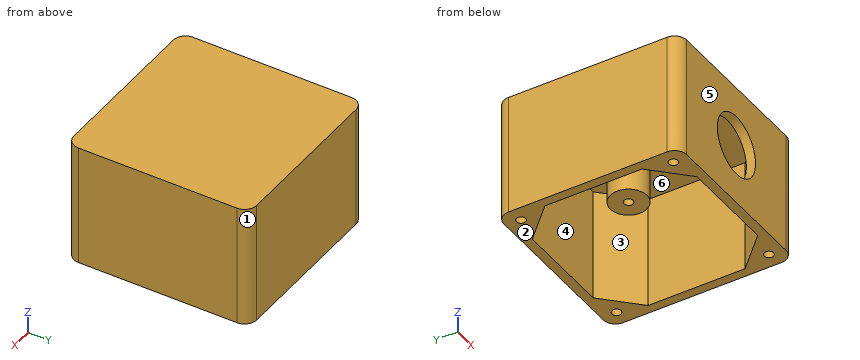
from build123d import *

# Parameters (mm, degrees)
SKETCH014_W     = 30
SKETCH014_H     = 30
PAD008_DEPTH    = 20
POCKET006_DEPTH = 18.5
SKETCH016_R     = 3
PAD009_DEPTH    = 6.5
SKETCH017_R     = 0.75
POCKET007_DEPTH = 5
SKETCH018_R     = 0.75
POCKET008_DEPTH = 15
SKETCH021_R     = 5
POCKET009_DEPTH = 5
FILLET001_R     = 2


with BuildPart() as part:
    # Sketch014 (on Face1 of ReferencePocket001) → Pad008 (new body)
    with BuildSketch(Plane(origin=(0, 0, 0), x_dir=(1, 0, 0), z_dir=(0, 0, -1))):
        with Locations((0, 2.9356231958)):
            Rectangle(SKETCH014_W, SKETCH014_H)
    extrude(amount=PAD008_DEPTH)

    # Sketch015 (on Face6 of Pad008) → Pocket006 (cut)
    with BuildSketch(Plane(origin=(0, 0, -20), x_dir=(1, 0, 0), z_dir=(0, 0, -1))):
        Polygon((-13.5, -5.0288428982), (-13.5, 10.9000892899), (-7.9644660941, 16.4356231958), (7.9644660941, 16.4356231958), (13.5, 10.9000892899), (13.5, -5.0288428982), (7.9644660941, -10.5643768042), (-7.9644660941, -10.5643768042), align=None)
    extrude(amount=-POCKET006_DEPTH, mode=Mode.SUBTRACT)

    # Sketch016 (on Face1 of ReferencePocket001) → Pad009 (join)
    with BuildSketch(Plane(origin=(0, 0, 0), x_dir=(1, 0, 0), z_dir=(0, 0, -1))):
        with Locations((-7, -4.15)):
            Circle(SKETCH016_R)
        with Locations((7, -4.15)):
            Circle(SKETCH016_R)
    extrude(amount=PAD009_DEPTH)

    # Sketch017 (on Face20 of Pad009) → Pocket007 (cut)
    with BuildSketch(Plane(origin=(0, 0, -6.5), x_dir=(1, 0, 0), z_dir=(0, 0, -1))):
        with Locations((-7, -4.15)):
            Circle(SKETCH017_R)
        with Locations((7, -4.15)):
            Circle(SKETCH017_R)
    extrude(amount=-POCKET007_DEPTH, mode=Mode.SUBTRACT)

    # Sketch018 (on Face5 of Pocket007) → Pocket008 (cut)
    with BuildSketch(Plane(origin=(0, 0, -20), x_dir=(1, 0, 0), z_dir=(0, 0, -1))):
        with Locations((-12.5, 15.4356231958)):
            Circle(SKETCH018_R)
        with Locations((12.5, 15.4356231958)):
            Circle(SKETCH018_R)
        with Locations((12.5, -9.5643768042)):
            Circle(SKETCH018_R)
        with Locations((-12.5, -9.5643768042)):
            Circle(SKETCH018_R)
    extrude(amount=-POCKET008_DEPTH, mode=Mode.SUBTRACT)

    # Sketch021 (on Face1 of Pocket008) → Pocket009 (cut)
    with BuildSketch(Plane.XZ.offset(17.9356231958)):
        with Locations((0, -10)):
            Circle(SKETCH021_R)
    extrude(amount=-POCKET009_DEPTH, mode=Mode.SUBTRACT)

    # Fillet001
    fillet001_edges = [part.edges().sort_by_distance(p)[0] for p in [
        (15, -17.935623, -10),
        (15, 12.064377, -10),
        (-15, -17.935623, -10),
        (-15, 12.064377, -10),
    ]]
    fillet(fillet001_edges, radius=FILLET001_R)


solid = part.part
Here's how the part is built. I have some questions about the finished solid (model axes, mm). Face numbers are marked on the shaded views. A direction names the side the tool comes from. Coordinates: 2 decimals unless noted, no trailing zeros. Write each loop counter-clockwise with the first axis right and the second up, starting at its lowest first coordinate (ties: lowest second). Pieces come first, ordered by that corner, then holes. Notation, with made-up numbers: (-13.5, -19) - (21.5, -19) arc R12 ccw to (21.5, 2) - close; hole circle Ø2 at (7.5, 88.5). An arc over 180 degrees is marked (long way). Use one line per item in the form item = value.
1) Thinking about a two-plate mould opening in Y: for the marked faces 1, 2, 3 and 4, which applies, released by +Y, released by -Y, zero draft, split by the parting line, or undercut?
Solved:
face_1 = released by +Y
face_2 = zero draft
face_3 = undercut
face_4 = undercut
2) Suppose I cut it at C-C, the plane z = -17.75. Write out the boundary of the cut face in (x, y), plus the area to 3 significant figures.
Solved:
outline = (-15, -15.94) arc R2 ccw to (-13, -17.94) - (13, -17.94) arc R2 ccw to (15, -15.94) - (15, 10.06) arc R2 ccw to (13, 12.06) - (-13, 12.06) arc R2 ccw to (-15, 10.06) - close; hole (-13.5, -10.9) - (-7.96, -16.44) - (7.96, -16.44) - (13.5, -10.9) - (13.5, 5.03) - (7.96, 10.56) - (-7.96, 10.56) - (-13.5, 5.03) - close; hole circle Ø1.5 at (-12.5, -15.44); hole circle Ø1.5 at (-12.5, 9.56); hole circle Ø1.5 at (12.5, -15.44); hole circle Ø1.5 at (12.5, 9.56)
area = 222 mm2
3) Suppose I cut it at D-D, the plane x = 7. Write out the boundary of the cut face in (y, z).
Solved:
outline = (-17.94, -20) - (-16.44, -20) - (-16.44, -1.5) - (1.15, -1.5) - (1.15, -6.5) - (3.4, -6.5) - (3.4, -1.5) - (4.9, -1.5) - (4.9, -6.5) - (7.15, -6.5) - (7.15, -1.5) - (10.56, -1.5) - (10.56, -20) - (12.06, -20) - (12.06, 0) - (-17.94, 0) - close
4) On a 3-axis mill with a long thin cutter (end or side, diameter ignored), from which of +Z, -Z, +X, -X, +Y, -Y can I reach the whole of each face in a straight line? I mean the marked faces 5 and 6. Say none if no direction works.
Solved:
face_5 = +Z, -Z, +X, -X, -Y
face_6 = -Z
5) Suppose I cut it at B-B, the plane y = 4.15. Write out the boundary of the cut face in (x, z), plus the area to 4 significant figures.
Solved:
outline = (-15, -20) - (-13.5, -20) - (-13.5, -1.5) - (-10, -1.5) - (-10, -6.5) - (-7.75, -6.5) - (-7.75, -1.5) - (-6.25, -1.5) - (-6.25, -6.5) - (-4, -6.5) - (-4, -1.5) - (4, -1.5) - (4, -6.5) - (6.25, -6.5) - (6.25, -1.5) - (7.75, -1.5) - (7.75, -6.5) - (10, -6.5) - (10, -1.5) - (13.5, -1.5) - (13.5, -20) - (15, -20) - (15, 0) - (-15, 0) - close
area = 145.5 mm2
6) I'm going to push flat-ended pins straight in: P1, Ø4, axis at x = -4.5, y = -9, coming from the -Z side; P2, Ø6.5, axis at x = 8.5, y = 3, coming from the -Z side. Where does each tip first touch, or does it pass through?
Solved:
P1 = -1.5
P2 = -6.5
7) Suppose I cut it at A-A, the plane x = 0. Write out the boundary of the cut face in (y, z), plus the area to 3 significant figures.
Solved:
outline = (-17.94, -20) - (-16.44, -20) - (-16.44, -15) - (-17.94, -15) - close; (-17.94, -5) - (-16.44, -5) - (-16.44, -1.5) - (10.56, -1.5) - (10.56, -20) - (12.06, -20) - (12.06, 0) - (-17.94, 0) - close
area = 85.5 mm2
8) I need wall thicknesses on line 1 (Y direction, x = -7, z = -3.7); line 2 (X direction, y = -9.75, z = -10.25); line 3 (Z direction, x = 0, y = -17.3). Which ranges of each line are inside material? Lowest first, please.
Solved:
line_1 = -17.94 to -16.44, 1.15 to 3.4, 4.9 to 7.15, 10.56 to 12.06
line_2 = -15 to -13.5, 13.5 to 15
line_3 = -20 to -15, -5 to 0
